```python
from build123d import *

# Parameters (mm, degrees)
SKETCH2_W                          = 63.5
SKETCH2_H                          = 31.75
BOSS_EXTRUDE1_DEPTH                = 31.75
F_59_64_0_92188_DIAMETER_HOLE1_D   = 23.415752
BOSS_EXTRUDE2_DEPTH                = 5.08
F_7_16_0_4375_DIAMETER_HOLE1_D     = 11.1125
F_7_16_0_4375_DIAMETER_HOLE1_DEPTH = 25.4
F_7_16_0_4375_DIAMETER_HOLE1_TIP   = 3.338531814


with BuildPart() as part:
    # Sketch2 → Boss-Extrude1 (new body)
    with BuildSketch(Plane(origin=(0, 0, 0), x_dir=(1, 0, 0), z_dir=(0, 1, 0))):
        Rectangle(SKETCH2_W, SKETCH2_H)
    extrude(amount=BOSS_EXTRUDE1_DEPTH)

    # 59/64 (0.92188) Diameter Hole1 (through all)
    with Locations(Plane(origin=(31.75, 0, 0), x_dir=(0, 0, -1), z_dir=(1, 0, 0))):
        with Locations((0, 15.875)):
            Hole(F_59_64_0_92188_DIAMETER_HOLE1_D / 2)

    # Sketch10 → Boss-Extrude2 (add)
    with BuildSketch(Plane.XY.offset(15.875)):
        Polygon((9.525, 11.1125), (-9.525, 20.6375), (-9.525, 6.35), (9.525, 6.35), align=None)
        Polygon((-9.525, 25.4), (-9.525, 20.6375), (9.525, 11.1125), (9.525, 25.4), align=None)
    extrude(amount=BOSS_EXTRUDE2_DEPTH)

    # 7/16 (0.4375) Diameter Hole1
    with Locations(Plane.XY.offset(20.955)):
        with Locations((0, 15.875)):
            Hole(F_7_16_0_4375_DIAMETER_HOLE1_D / 2, depth=F_7_16_0_4375_DIAMETER_HOLE1_DEPTH)
            with Locations((0, 0, -(F_7_16_0_4375_DIAMETER_HOLE1_DEPTH + F_7_16_0_4375_DIAMETER_HOLE1_TIP / 2))):  # 118° drill point
                Cone(0, F_7_16_0_4375_DIAMETER_HOLE1_D / 2, F_7_16_0_4375_DIAMETER_HOLE1_TIP, mode=Mode.SUBTRACT)


solid = part.part
```
Verification items for the finished model (mm, model axes). A direction names the side the tool comes from. Round coordinates to 2 decimals unless told otherwise and drop trailing zeros. Loops run counter-clockwise (first coordinate to the right, second up) from the corner with the lowest first, then second, coordinate; pieces in that order, holes last. Notation, with made-up numbers: (27, 16) -> (57, 16) arc R22 cw to (57, 40) -> close; hole circle Ø4 at (10, -14). An arc over 180 degrees is marked (long way). Answer as a JSON object with one key per item and string values.
Q1. Access from +Z, -Z, +X, -X, +Y, -Y to the whole of each face (thin tool, end or side, straight path). Record for faces 1 (the flat face through (0, 25.4, 18)), 2 (the flat face through (9.525, 16, 18)), 3 (the flat face through (0, 6.35, 18)).
Data:
{"face 1": "+Z, +X, -X, +Y", "face 2": "+Z, +X, +Y, -Y", "face 3": "+Z, +X, -X, -Y"}
Q2. Draft check along Y on faces 4 (the flat face through (0, 31.75, 0)), 5 (the cylindrical face through (-0.445, 16.39, -11.697)), 6 (the flat face through (0, 0, 0)). Enter one of: pulls with the +Y half, pulls with the -Y half, needs draft (parallel to the pull), parting line crosses it, or undercut.
Data:
{"face 4": "pulls with the +Y half", "face 5": "undercut", "face 6": "pulls with the -Y half"}
Q3. Section check B-B (x = 25.5). Record the boundary of the cut face in (y, z) (3 decimals).
Data:
{"outline": "(0, -15.875) -> (31.75, -15.875) -> (31.75, 15.875) -> (0, 15.875) -> close; hole circle Ø23.416 at (15.875, 0)"}
Q4. Scan lines: line 1 (Y direction, x = -1, z = 0); line 2 (X direction, y = 16, z = 14); line 3 (Y direction, x = 0, z = 18). Record each from-to range of solid material in increasing order. Write a range as from..to.
Data:
{"line 1": "y = 0..4.17, 27.58..31.75", "line 2": "x = -31.75..-5.55, 5.55..31.75", "line 3": "y = 6.35..10.32, 21.43..25.4"}
Q5. Go/stop test with flat-tipped pins: P1, Ø2.5, axis at y = 13.5, z = 17.5, coming from the -X side (3 decimals); P2, Ø4, axis at x = -2, z = 17, coming from the +Y side; P3, Ø18.5, axis at y = 15.875, z = 0, coming from the +X side; P4, Ø5, axis at x = 24, y = 18, coming from the +Z side (3 decimals). Record where each tip stops, or that it passes through.
Data:
{"P1": "stops at x = -9.525", "P2": "stops at y = 31.75", "P3": "passes through", "P4": "stops at z = 15.875"}
Q6. Section check D-D (x = 0). Record the boundary of the cut face in (y, z) (3 decimals).
Data:
{"outline": "(0, -15.875) -> (31.75, -15.875) -> (31.75, 15.875) -> (25.4, 15.875) -> (25.4, 20.955) -> (21.431, 20.955) -> (21.431, 10.305) arc R11.708 cw (long way) to (10.319, 10.305) -> (10.319, 20.955) -> (6.35, 20.955) -> (6.35, 15.875) -> (0, 15.875) -> close"}
Q7. Section check C-C (y = 23). Record the boundary of the cut face in (x, z) (3 decimals).
Data:
{"outline": "(-31.75, -15.875) -> (31.75, -15.875) -> (31.75, -9.29) -> (-31.75, -9.29) -> close; (-31.75, 9.29) -> (31.75, 9.29) -> (31.75, 15.875) -> (9.525, 15.875) -> (9.525, 20.955) -> (-9.525, 20.955) -> (-9.525, 15.875) -> (-31.75, 15.875) -> close"}
Q8. Section check A-A (z = 0). Record the boundary of the cut face in (x, y).
Data:
{"outline": "(-31.75, 0) -> (31.75, 0) -> (31.75, 4.17) -> (-31.75, 4.17) -> close; (-31.75, 27.58) -> (31.75, 27.58) -> (31.75, 31.75) -> (-31.75, 31.75) -> close"}
